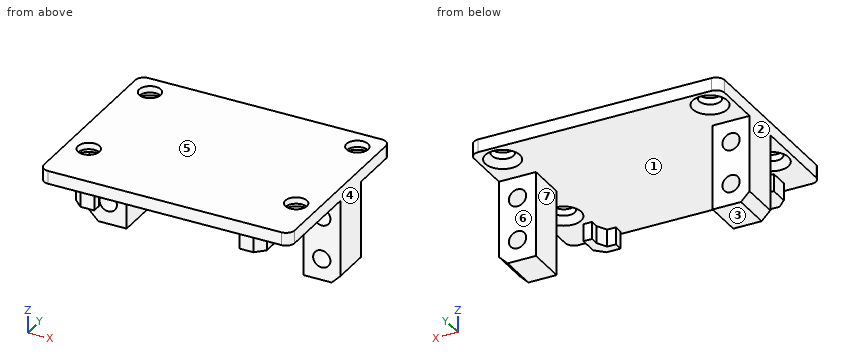
Autodesk Inventor part; units mm, degrees
ref_plane "YZ Plane" through (0, 0, 0) normal (1, 0, 0) x (0, 1, 0)
ref_plane "XZ Plane" through (0, 0, 0) normal (0, 1, 0) x (-1, 0, 0)
ref_plane "XY Plane" through (0, 0, 0) normal (0, 0, 1) x (1, 0, 0)
sketch "Sketch1" plane through (0, 0, 0) normal (0, 0, 1) x (1, 0, 0)
  line L0 (-29, 12.3) -> (29, 12.3)
  line L1 (29, 12.3) -> (29, -31.3)
  line L2 (29, -31.3) -> (-29, -31.3)
  line L3 (-29, -31.3) -> (-29, 12.3)
  line L4 (-15.4526, -28.3) -> (15.4526, -28.3) construction
  line L5 (-27, 2.4) -> (-27, 0) construction
  line L6 (15.475, 12.3) -> (4.725, 12.3) construction
  point P0 (0, 12.3)
  point P1 (0, -31.3)
  point P2 (0, 0)
  point P3 (10.1, 12.3)
  dimension "MotorMountBaseBracketOffset" = 2
  dimension "MotorMountBaseBottomOffset" = 3
extrude "Extrusion1" add sketch "Sketch1" along normal blind 3
sketch "Sketch2" plane through (0, 0, 0) normal (0, 0, -1) x (-1, 0, 0)
  line L0 (-29, -31.3) -> (-29, 12.3) construction
  line L1 (-26, 0) -> (-19.25, 0) construction
  line L2 (-19.95, -21.3) -> (-19.95, -0.5) construction
  line L3 (-29, -9.5) -> (-20.45, -9.5)
  line L4 (-20.45, -9.5) -> (-20.45, -0.5)
  line L5 (-20.45, -0.5) -> (-29, -0.5)
  line L6 (-29, -0.5) -> (-29, -9.5)
  dimension "d66" = 9
  dimension "d67" = 0.5
  dimension "d68" = 0.5
extrude "Extrusion6" add sketch "Sketch2" along normal blind 19.7
sketch "Sketch7" plane through (0, 0, 0) normal (0, 0, -1) x (-1, 0, 0)
  line L0 (-16.8094, -28.4) -> (-16.8094, -30.4)
  line L1 (-18.8094, -28.4) -> (-16.8094, -28.4)
  line L2 (-20.05, -26.1255) -> (-18.8094, -28.4)
  line L3 (-20.05, -24.1255) -> (-20.05, -26.1255)
  line L4 (-22.05, -24.1255) -> (-20.05, -24.1255)
  line L5 (-22.05, -30.4) -> (-22.05, -24.1255)
  line L6 (-16.8094, -30.4) -> (-22.05, -30.4)
  line L7 (15.4526, -28.3) -> (-15.4526, -28.3) construction
  line L8 (-19.35, -27.2) -> (-18.75, -28.3) construction
  line L9 (-19.95, -21.3) -> (-19.95, -0.5) construction
  point P0 (0, 0)
  dimension "d79" = 2
  dimension "d82" = 0.1
  dimension "d83" = 0.1
  dimension "d84" = 0.1
extrude "Extrusion7" add sketch "Sketch7" along normal blind 4
sketch "Sketch5" plane through (0, 0, 0) normal (0, 0, -1) x (-1, 0, 0)
  circle A0 centre (-24, 7.3) radius 2.5
  circle A1 centre (-24, -19.3) radius 2.5
  point P0 (0, 0)
  point P1 (-29, -31.3)
  point P2 (-29, 12.3)
  dimension "d89" = 5
  dimension "d90" = 5
  dimension "d91" = 5
  dimension "MotorMountBottomHoleOffset" = 12
extrude "Extrusion4" cut sketch "Sketch5" against normal through all
chamfer "Chamfer1" distance 1.5 angle 45 2 edges at (26.5, 7.3, 0) (26.5, -19.3, 0)
chamfer "Chamfer4" distance 2 angle 45 2 edges at (29, -5, -19.7) (22.05, -30.4, -2)
sketch "Sketch8" plane through (20.45, -0.5, 0) normal (0, 1, 0) x (1, 0, 0)
  arc A0 (5.9164, 6.2173) -> (5.9164, 3.6327) centre (4.2611, 4.925) ccw construction
  arc A1 (5.9164, 16.0673) -> (5.9164, 13.4827) centre (4.2611, 14.775) ccw construction
  circle A2 centre (4.2611, 14.775) radius 2
  circle A3 centre (4.2611, 4.925) radius 2
  point P0 (-20.45, 0)
  dimension "MotorMountPillarHoleDia" = 4
  dimension "d99" = 4
extrude "Extrusion8" cut sketch "Sketch8" against normal through all
mirror "Mirror1" about plane through (0, 0, 0) normal (1, 0, 0) of "Extrusion7", "Extrusion4", "Chamfer1", "Extrusion6", "Chamfer4", "Extrusion8"
fillet "Fillet1" radius 2 4 edges at (29, -31.3, 1.5) (29, 12.3, 1.5) (-29, 12.3, 1.5) (-29, -31.3, 1.5)
equation "\"d66\" = MotorMountPillarDepth"
equation "\"d67\" = MotorMountPillarOffset"
equation "\"d68\" = MotorMountPillarOffset"
equation "\"d82\" = MotorMountLocatorOffset"
equation "\"d83\" = MotorMountLocatorOffset"
equation "\"d84\" = MotorMountLocatorOffset"
equation "\"d89\" = ScrewHoleDia"
equation "\"d42\" = ScrewHoleFillet"
equation "\"d99\" = MotorMountPillarHoleDia"
properties part number "MotorCasingSmall"
Input: part model. Units: mm. Frame: model coordinates. Face numbers are marked on the shaded views. A direction names the side the tool comes from. Round coordinates to 2 decimals unless told otherwise and drop trailing zeros. Write each loop counter-clockwise with the first axis right and the second up, starting at its lowest first coordinate (ties: lowest second). Pieces come first, ordered by that corner, then holes.
1) Reachability of the marked faces 5, 6 and 7 from +Z, -Z, +X, -X, +Y, -Y: full face, straight path, thin tool, end or side. Return the list, or none.
2) Cut plane A-A (y = 7.3). Return the cut outline in (x, z).
3) Cut plane C-C (x = 24). Return the cut outline in (y, z), then the cut area to 3 significant figures.
4) Cut plane D-D (x = 4.5). Return the cut outline in (y, z), then the cut area to 3 significant figures.
5) Cut plane B-B (z = -8.25). Return the cut outline in (x, y), then the cut area to 3 significant figures.
6) Ray query, L1, parallel to X at y = -3, z = -11; L2, parallel to X at y = -7.5, z = -13.5; L3, parallel to Z at x = -14, y = 0.5. Return the intervals inside material, ascending.
7) Draft query along X for the marked faces 1, 2, 3 and 4. Return one class per face: pulls with the +X half, pulls with the -X half, needs draft (parallel to the pull), parting line crosses it, or undercut.
8) Contact query for flat-ended pins moving along their axis: P1, Ø1, axis at x = -21.5, z = -3, coming from the +Y side; P2, Ø3, axis at x = -15, y = -9.5, coming from the -Z side; P3, Ø4, axis at x = 24, y = -19.3, coming from the +Z side; P4, Ø0.6, axis at y = -25, z = -1.5, coming from the +X side. Output: stop coordinate, or through.
Geometry says:
1. face 5: +Z, +X, -X, +Y, -Y
1. face 6: -Z, +X, -X, +Y
1. face 7: -Z, +Y
2. outline: (-29, 0) - (-28, 0) - (-26.5, 1.5) - (-26.5, 3) - (-29, 3) - close; (-21.5, 1.5) - (-20, 0) - (20, 0) - (21.5, 1.5) - (21.5, 3) - (-21.5, 3) - close; (26.5, 1.5) - (28, 0) - (29, 0) - (29, 3) - (26.5, 3) - close
3. outline: (-31.3, 0) - (-23.3, 0) - (-21.8, 1.5) - (-21.8, 3) - (-31.3, 3) - close; (-16.8, 1.5) - (-15.3, 0) - (-9.5, 0) - (-9.5, -3.06) - (-0.5, -3.06) - (-0.5, 0) - (3.3, 0) - (4.8, 1.5) - (4.8, 3) - (-16.8, 3) - close; (-9.5, -19.7) - (-0.5, -19.7) - (-0.5, -16.64) - (-9.5, -16.64) - close; (-9.5, -12.91) - (-0.5, -12.91) - (-0.5, -6.79) - (-9.5, -6.79) - close; (9.8, 1.5) - (11.3, 0) - (12.3, 0) - (12.3, 3) - (9.8, 3) - close
3. area: 206 mm2
4. outline: (-31.3, 0) - (12.3, 0) - (12.3, 3) - (-31.3, 3) - close
4. area: 131 mm2
5. outline: (-29, -9.5) - (-20.45, -9.5) - (-20.45, -0.5) - (-29, -0.5) - close; (20.45, -9.5) - (29, -9.5) - (29, -0.5) - (20.45, -0.5) - close
5. area: 154 mm2
6. L1: x = -29 to -20.45, 20.45 to 29
6. L2: x = -29 to -26.25, -23.17 to -20.45, 20.45 to 23.17, 26.25 to 29
6. L3: z = 0 to 3
7. face 1: undercut
7. face 2: pulls with the -X half
7. face 3: needs draft
7. face 4: pulls with the +X half
8. P1: stops at y = -0.5
8. P2: stops at z = 0
8. P3: passes through
8. P4: stops at x = 22.05
